Geometry: final body of the model. Coordinates: model frame, mm. Face numbers are marked on the shaded views. A direction names the side the tool comes from. Round coordinates to 2 decimals unless told otherwise and drop trailing zeros. Loops run counter-clockwise (first coordinate to the right, second up) from the corner with the lowest first, then second, coordinate; pieces in that order, holes last. Notation, with made-up numbers: M 38.25,34 L 91.25,34 A17 cw 91.25,57 Z; hole C 40,83.5 d7. An arc over 180 degrees is marked long. Answer as a JSON object with one key per item and string values.
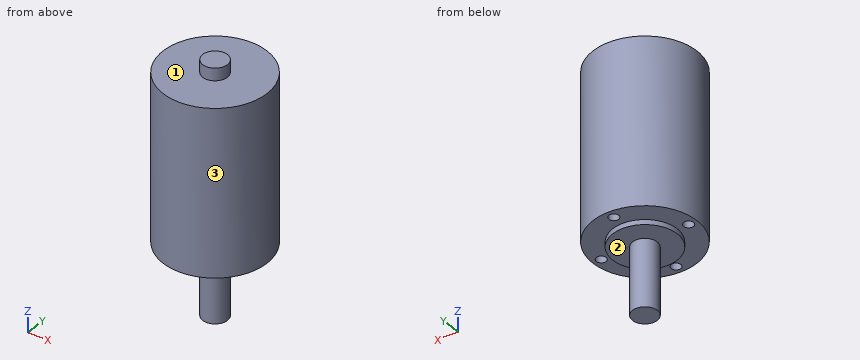
from build123d import *

# Parameters (mm, degrees)
SKETCH_1_R          = 21
EXTRUDE_1_DEPTH     = 67
SKETCH_3_R          = 13
EXTRUDE_3_DEPTH     = 2
SKETCH_4_R          = 5
EXTRUDE_4_DEPTH     = 29
SKETCH_5_R          = 2.016017639
SKETCH_5_R_2        = 2.040158569
SKETCH_5_R_3        = 1.937096917
SKETCH_5_R_4        = 2
SKETCH_5_R_5        = 4.5
EXTRUDE_5_DEPTH     = 0.7
EXTRUDE_START       = 5
SKETCH_7_R          = 5
EXTRUDE_6_DEPTH     = 5
SKETCH_6_R          = 2
CUT_EXTRUDE_1_DEPTH = 7


with BuildPart() as part:
    # 草图1 → 凸台-拉伸1 (new body)
    with BuildSketch(Plane.XY):
        Circle(SKETCH_1_R)
    extrude(amount=EXTRUDE_1_DEPTH)

    # 草图3 → 凸台-拉伸3 (add)
    with BuildSketch(Plane.XY):
        Circle(SKETCH_3_R)
    extrude(amount=-EXTRUDE_3_DEPTH)

    # 草图4 → 凸台-拉伸4 (add)
    with BuildSketch(Plane.XY):
        Circle(SKETCH_4_R)
    extrude(amount=-EXTRUDE_4_DEPTH)

    # 草图5 → 凸台-拉伸5 (add)
    with BuildSketch(Plane.XY):
        with Locations((17.5, 0)):
            Circle(SKETCH_5_R)
        with Locations((0, -17.5)):
            Circle(SKETCH_5_R_2)
        with Locations((-17.5, 0)):
            Circle(SKETCH_5_R_3)
        with Locations((0, 17.5)):
            Circle(SKETCH_5_R_4)
        with Locations((12.557158291, 12.188838159)):
            Circle(SKETCH_5_R_4)
        with Locations((-12.557158291, 12.188838159)):
            Circle(SKETCH_5_R_4)
        with Locations((-12.557158291, -12.188838159)):
            Circle(SKETCH_5_R_4)
        with Locations((12.557158291, -12.188838159)):
            Circle(SKETCH_5_R_4)
        Circle(SKETCH_5_R_5)
    extrude(amount=EXTRUDE_5_DEPTH)

    # 草图7 → 凸台-拉伸6 (add)
    with BuildSketch(Plane.XY.offset(67).offset(EXTRUDE_START)):
        Circle(SKETCH_7_R)
    extrude(amount=-EXTRUDE_6_DEPTH)

    # 草图6 → 切除-拉伸1 (cut)
    with BuildSketch(Plane.XY):
        with Locations((-17.5, 0)):
            Circle(SKETCH_6_R)
        with Locations((17.5, 0)):
            Circle(SKETCH_6_R)
        with Locations((0, 17.5)):
            Circle(SKETCH_6_R)
        with Locations((0, -17.5)):
            Circle(SKETCH_6_R)
    extrude(amount=CUT_EXTRUDE_1_DEPTH, mode=Mode.SUBTRACT)


solid = part.part
1) Ray query, line 1 (Y direction, x = 0, z = 2.5); line 2 (Z direction, x = -13.5, y = -8.5); line 3 (Z direction, x = -10, y = -4). Return the intervals inside material, ascending.
Results:
{"line 1": "-21 to -19.5, -15.5 to 15.5, 19.5 to 21", "line 2": "0 to 67", "line 3": "-2 to 67"}
2) Reachability of the marked faces 1, 2 and 3 from +Z, -Z, +X, -X, +Y, -Y: full face, straight path, thin tool, end or side. Return the list, or none.
Results:
{"face 1": "+Z", "face 2": "-Z", "face 3": "+Z, -Z"}
3) Section query D-D (y = -7.5). Return the cut outline in (x, z).
Results:
{"outline": "M -19.62,0 L -10.62,0 L -10.62,-2 L 10.62,-2 L 10.62,0 L 19.62,0 L 19.62,67 L -19.62,67 Z"}
4) Section query C-C (z = -9.5). Return the cut outline in (x, y).
Results:
{"outline": "C 0,0 d10"}
5) Pin query (flat end, axial travel): P1, Ø4.5, axis at x = 0, y = 17, coming from the -Z side; P2, Ø3, axis at x = 15.5, z = 9, coming from the -Y side; P3, Ø5, axis at x = -17.5, y = 0, coming from the +Z side. Return the tip coordinate at first contact, or that it passes through.
Results:
{"P1": "z = 0", "P2": "y = -15.65", "P3": "z = 67"}
6) Section query A-A (y = 1). Return the cut outline in (x, z), and give its area (3 significant figures).
Results:
{"outline": "M -20.98,0 L -19.23,0 L -19.23,7 L -15.77,7 L -15.77,0 L -12.96,0 L -12.96,-2 L -4.9,-2 L -4.9,-29 L 4.9,-29 L 4.9,-2 L 12.96,-2 L 12.96,0 L 15.77,0 L 15.77,7 L 19.23,7 L 19.23,0 L 20.98,0 L 20.98,67 L 4.9,67 L 4.9,72 L -4.9,72 L -4.9,67 L -20.98,67 Z", "area": "3,130 mm2"}
7) Section query B-B (x = -17.5). Return the cut outline in (y, z), and give its area (3 significant figures).
Results:
{"outline": "M -11.61,0 L -2,0 L -2,7 L 2,7 L 2,0 L 11.61,0 L 11.61,67 L -11.61,67 Z", "area": "1,530 mm2"}
